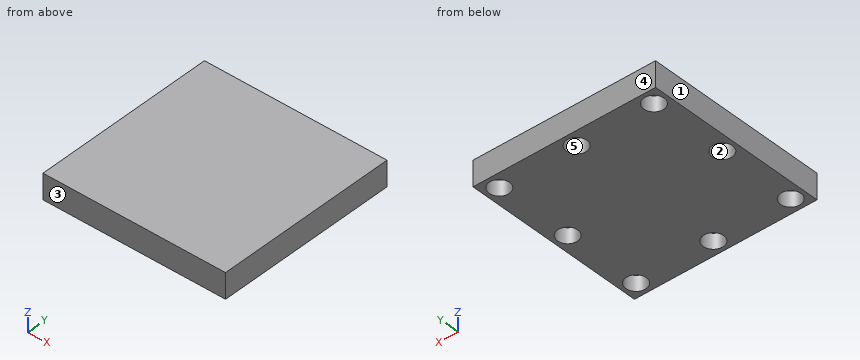
from build123d import *

# Parameters (mm, degrees)
SKETCH_1_W      = 36
SKETCH_1_H      = 36
SKETCH_1_R      = 2
EXTRUDE_1_DEPTH = 3
SKETCH_2_W      = 36
SKETCH_2_H      = 36
EXTRUDE_2_DEPTH = 2


with BuildPart() as part:
    # 스케치1 → 보스-돌출1 (new body)
    with BuildSketch(Plane.XY):
        with Locations((17.845923561, -15.757575758)):
            Rectangle(SKETCH_1_W, SKETCH_1_H)
        with Locations((2.595923561, -0.507575758)):
            Circle(SKETCH_1_R, mode=Mode.SUBTRACT)
        with Locations((17.845923561, -0.507575758)):
            Circle(SKETCH_1_R, mode=Mode.SUBTRACT)
        with Locations((33.095923561, -0.507575758)):
            Circle(SKETCH_1_R, mode=Mode.SUBTRACT)
        with Locations((33.095923561, -15.757575758)):
            Circle(SKETCH_1_R, mode=Mode.SUBTRACT)
        with Locations((33.095923561, -31.007575758)):
            Circle(SKETCH_1_R, mode=Mode.SUBTRACT)
        with Locations((17.845923561, -31.007575758)):
            Circle(SKETCH_1_R, mode=Mode.SUBTRACT)
        with Locations((2.595923561, -31.007575758)):
            Circle(SKETCH_1_R, mode=Mode.SUBTRACT)
        with Locations((2.595923561, -15.757575758)):
            Circle(SKETCH_1_R, mode=Mode.SUBTRACT)
    extrude(amount=EXTRUDE_1_DEPTH)

    # 스케치2 → 보스-돌출2 (add)
    with BuildSketch(Plane.XY.offset(3)):
        with Locations((17.845923561, -15.757575758)):
            Rectangle(SKETCH_2_W, SKETCH_2_H)
    extrude(amount=EXTRUDE_2_DEPTH)


solid = part.part
The model under review builds one solid part; all positions refer to its coordinate system, in mm. Face numbers are marked on the shaded views. A direction names the side the tool comes from. Coordinates: 2 decimals unless noted, no trailing zeros. Write each loop counter-clockwise with the first axis right and the second up, starting at its lowest first coordinate (ties: lowest second). Pieces come first, ordered by that corner, then holes. Notation, with made-up numbers: (-22.75, 0) - (12.25, 0) arc R8 cw to (12.25, 10) - close; hole circle Ø8 at (16.5, 20.25). An arc over 180 degrees is marked (long way). Answer as a JSON object with one key per item and string values. Group by question number.
1. Add section C-C (y = -29.5). Give the boundary of the cut face in (x, z), plus the area to 3 significant figures.
2. Add section D-D (y = -14.5). Give the boundary of the cut face in (x, z).
3. Add section A-A (z = 1.65). Give the number of separate pieces and of enclosed holes in the cut face, plus the area to 3 significant figures.
4. Clearance check with a flat-ended pin moving along its axis: pin 1 Ø3 at (x, y) = (18, -31) entering from -Z. State where the tip first meets the part, or that it passes through.
5. Add section B-B (x = 18). Give the boundary of the cut face in (y, z).
6. Machinability: for the marked faces 1 and 2, which of the approach directions +Z, -Z, +X, -X, +Y, -Y give a long, thin tool a straight path to every point of the face, cutting with its end or side? Answer none if there is none.
7. To check wall thickness, follow probe 1 along Y at (x, z) = (17.5, 0.75); probe 2 along X at (y, z) = (-1, 2.5); probe 3 along X at (y, z) = (-2, 2.4). State the ranges of each line that lie inside material, in increasing order.
8. Mouldability with a two-part tool opening along Y and no side actions: class the marked faces 3, 4 and 5 as pulls with the +Y half, pulls with the -Y half, needs draft (parallel to the pull), parting line crosses it, or undercut.
Findings:
{
 "1": {"outline": "(-0.15, 0) - (1.28, 0) - (1.28, 3) - (3.91, 3) - (3.91, 0) - (16.53, 0) - (16.53, 3) - (19.16, 3) - (19.16, 0) - (31.78, 0) - (31.78, 3) - (34.41, 3) - (34.41, 0) - (35.85, 0) - (35.85, 5) - (-0.15, 5) - close", "area": "156 mm²"},
 "2": {"outline": "(-0.15, 0) - (1.04, 0) - (1.04, 3) - (4.15, 3) - (4.15, 0) - (31.54, 0) - (31.54, 3) - (34.65, 3) - (34.65, 0) - (35.85, 0) - (35.85, 5) - (-0.15, 5) - close"},
 "3": {"separate pieces": "1", "enclosed holes": "8", "area": "1,200 mm²"},
 "4": {"pin 1": "z = 3"},
 "5": {"outline": "(-33.76, 0) - (-33, 0) - (-33, 3) - (-29.01, 3) - (-29.01, 0) - (-2.5, 0) - (-2.5, 3) - (1.49, 3) - (1.49, 0) - (2.24, 0) - (2.24, 5) - (-33.76, 5) - close"},
 "6": {"face 1": "+Z, -Z, -X, +Y, -Y", "face 2": "-Z"},
 "7": {"probe 1": "-33.76 to -32.98, -29.04 to -2.48, 1.46 to 2.24", "probe 2": "-0.15 to 0.66, 4.53 to 15.91, 19.78 to 31.16, 35.03 to 35.85", "probe 3": "-0.15 to 1.26, 3.93 to 16.51, 19.18 to 31.76, 34.43 to 35.85"},
 "8": {"face 3": "pulls with the -Y half", "face 4": "pulls with the +Y half", "face 5": "undercut"}
}
